Here's the drawing with two shaded views (mm, measured from the low corner). I have some questions. A direction names the side the tool comes from. Coordinates: 2 decimals unless noted, no trailing zeros. Write each loop counter-clockwise with the first axis right and the second up, starting at its lowest first coordinate (ties: lowest second). Pieces come first, ordered by that corner, then holes.
Item 1: We'd pull the mould along Y, two halves only. Please class the marked faces 4, 5 and 6: +Y half, -Y half, draft (parallel to the pull), parting line (faces both ways), or undercut.
Item 2: For the marked faces 1, 2 and 3, which set-ups out of +Z, -Z, +X, -X, +Y, -Y let a thin tool reach every point of the face, with its end or its side?
Item 3: If we section it at D-D (y = 78): Please give me the cut outline in (x, z).
Item 4: If I drill on line 1 (X direction, y = 6.35, z = 11.5); line 2 (Y direction, x = 33.5, z = 15); line 3 (Y direction, x = 134.5, z = 8.25), over which ranges is the centre line in solid material (lowest first)?
Item 5: If we section it at A-A (z = 16): Count the separate pieces of the cut face and the enclosed holes in it, then the cut area to 3 significant figures.
Item 6: If we section it at B-B (x = 127): Please give me the cut outline in (y, z).
Item 7: I'm going to push flat-ended pins straight in: pin 1 Ø7.5 at (x, y) = (64, 57) entering from +Z; pin 2 Ø6 at (y, z) = (24.5, 17) entering from -X; pin 3 Ø1.5 at (x, y) = (73, 31.5) entering from +Z; pin 4 Ø3 at (x, y) = (101.6, 95.25) entering from +Z. Where does each tip first touch, or does it pass through?
Item 8: If we section it at C-C (y = 95.25): Please give me the cut outline in (x, z), then the cut area to 3 significant figures.
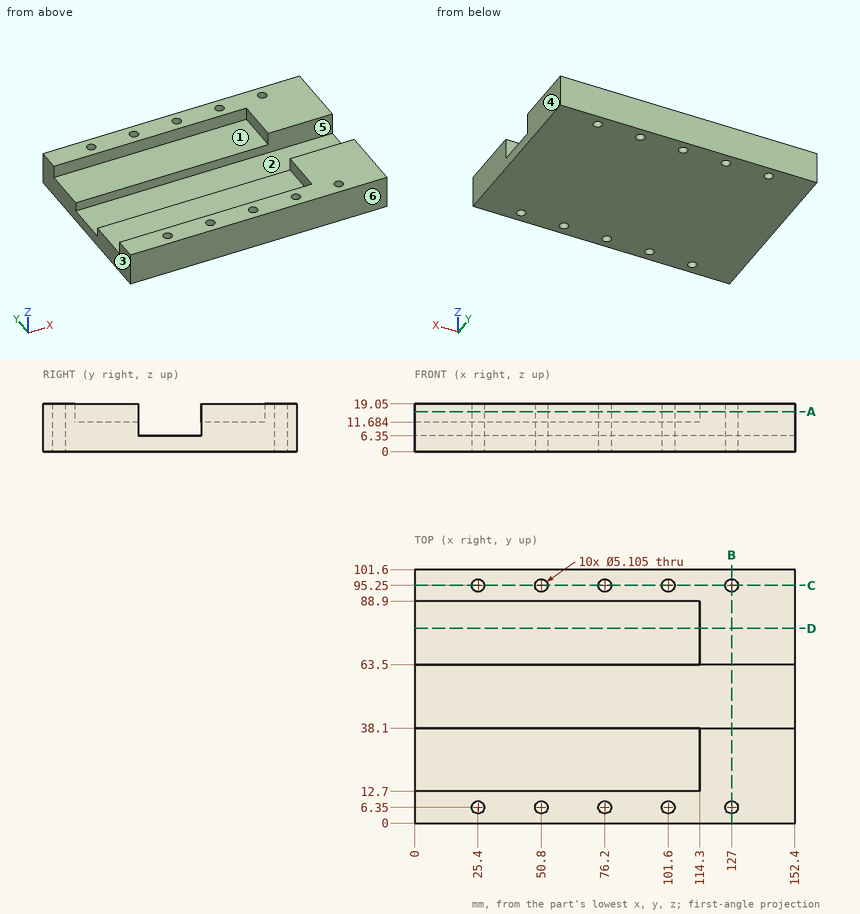
Answer list:
1. face 4: draft
1. face 5: undercut
1. face 6: -Y half
2. face 1: +Z, -X
2. face 2: +Z, +X, -X
2. face 3: +Z, -Z, -X, +Y, -Y
3. outline: (0, 0) - (152.4, 0) - (152.4, 19.05) - (114.3, 19.05) - (114.3, 11.68) - (0, 11.68) - close
4. line 1: x = 0 to 22.85, 27.95 to 48.25, 53.35 to 73.65, 78.75 to 99.05, 104.15 to 124.45, 129.55 to 152.4
4. line 2: y = 0 to 12.7, 88.9 to 101.6
4. line 3: y = 0 to 38.1, 63.5 to 101.6
5. separate pieces: 2
5. enclosed holes: 10
5. area: 5,600 mm2
6. outline: (0, 0) - (3.8, 0) - (3.8, 19.05) - (0, 19.05) - close; (8.9, 0) - (92.7, 0) - (92.7, 19.05) - (63.5, 19.05) - (63.5, 6.35) - (38.1, 6.35) - (38.1, 19.05) - (8.9, 19.05) - close; (97.8, 0) - (101.6, 0) - (101.6, 19.05) - (97.8, 19.05) - close
7. pin 1: stops at z = 6.35
7. pin 2: stops at x = 114.3
7. pin 3: stops at z = 11.68
7. pin 4: passes through
8. outline: (0, 0) - (22.85, 0) - (22.85, 19.05) - (0, 19.05) - close; (27.95, 0) - (48.25, 0) - (48.25, 19.05) - (27.95, 19.05) - close; (53.35, 0) - (73.65, 0) - (73.65, 19.05) - (53.35, 19.05) - close; (78.75, 0) - (99.05, 0) - (99.05, 19.05) - (78.75, 19.05) - close; (104.15, 0) - (124.45, 0) - (124.45, 19.05) - (104.15, 19.05) - close; (129.55, 0) - (152.4, 0) - (152.4, 19.05) - (129.55, 19.05) - close
8. area: 2,420 mm2
